Work out the finished part from the listing and answer in its coordinate system (mm). A direction names the side the tool comes from. Give positions to 0.01 mm unless a question says otherwise; leave off trailing zeros. Loops run counter-clockwise (first coordinate to the right, second up) from the corner with the lowest first, then second, coordinate; pieces in that order, holes last. Notation, with made-up numbers: (-6, 69) - (20, 69) arc R25 cw to (20, 81) - close; hole circle Ø8 at (-39.5, -10.75). An arc over 180 degrees is marked (long way). One line per question, with ' | ' between items.
Autodesk Inventor part; units mm, degrees
ref_plane "YZ Plane" through (0, 0, 0) normal (1, 0, 0) x (0, 1, 0)
ref_plane "XZ Plane" through (0, 0, 0) normal (0, 1, 0) x (-1, 0, 0)
ref_plane "XY Plane" through (0, 0, 0) normal (0, 0, 1) x (1, 0, 0)
sketch "Sketch1" plane through (0, 0, 0) normal (0, 0, 1) x (1, 0, 0)
  line L0 (90.4273, 0.002) -> (0, 0.002)
  line L1 (0, 0.002) -> (0, -88.6441)
  arc A0 (0, -88.6441) -> (7.9382, -98.4293) centre (10, -88.6441) ccw
  arc A1 (16.0457, -111.012) -> (7.9382, -98.4293) centre (6.4076, -108.3189) ccw
  arc A2 (145.7944, -114.2869) -> (148.0953, -110.4201) centre (146.9707, -112.3688) ccw
  circle A3 centre (97.4707, -122.3689) radius 2.25
  circle A4 centre (97.4707, -112.3689) radius 2.25
  circle A5 centre (78.1758, -122.3689) radius 2.25
  arc A6 (145.7944, -124.2869) -> (148.0953, -120.4201) centre (146.9707, -122.3689) ccw
  circle A7 centre (22.6171, -8.5119) radius 2.8
  circle A8 centre (22.6171, -40.5119) radius 2.8
  circle A9 centre (28.6758, -122.3689) radius 2.25
  circle A10 centre (28.6758, -112.3689) radius 2.25
  circle A11 centre (78.1758, -112.3689) radius 2.25
  circle A12 centre (78.9344, -21.998) radius 3.25
  circle A13 centre (10, -90.6616) radius 3.3
  line L2 (73.0605, -128.2915) -> (33.527, -128.2915)
  arc A14 (32.527, -127.2915) -> (33.527, -128.2915) centre (33.527, -127.2915) ccw
  line L3 (32.527, -127.2915) -> (32.527, -107.4915)
  arc A15 (33.527, -106.4915) -> (32.527, -107.4915) centre (33.527, -107.4915) ccw
  line L4 (33.527, -106.4915) -> (73.0605, -106.4915)
  arc A16 (74.0605, -107.4915) -> (73.0605, -106.4915) centre (73.0605, -107.4915) ccw
  line L5 (74.0605, -107.4915) -> (74.0605, -127.2915)
  arc A17 (73.0605, -128.2915) -> (74.0605, -127.2915) centre (73.0605, -127.2915) ccw
  line L6 (142.1195, -128.2915) -> (102.586, -128.2915)
  arc A18 (101.586, -127.2915) -> (102.586, -128.2915) centre (102.586, -127.2915) ccw
  line L7 (101.586, -127.2915) -> (101.586, -107.4915)
  arc A19 (102.586, -106.4915) -> (101.586, -107.4915) centre (102.586, -107.4915) ccw
  line L8 (102.586, -106.4915) -> (142.1195, -106.4915)
  arc A20 (143.1195, -107.4915) -> (142.1195, -106.4915) centre (142.1195, -107.4915) ccw
  line L9 (143.1195, -107.4915) -> (143.1195, -127.2915)
  arc A21 (142.1195, -128.2915) -> (143.1195, -127.2915) centre (142.1195, -127.2915) ccw
  circle A22 centre (146.9707, -112.3688) radius 2.25
  circle A23 centre (146.9707, -122.3689) radius 2.25
  line L10 (28.6758, -112.3689) -> (146.9707, -112.3688) construction
  line L11 (28.6758, -122.3689) -> (146.9707, -122.3689) construction
  circle A24 centre (43.3732, -117.3689) radius 5.9 construction
  circle A25 centre (132.2732, -117.3688) radius 5.9 construction
  circle A26 centre (43.3732, -117.3689) radius 6
  circle A27 centre (132.2732, -117.3688) radius 6
  line L12 (10, -90.6616) -> (176.2125, -90.6616) construction
  circle A28 centre (78.9344, -21.998) radius 6
  circle A29 centre (79.375, -41.275) radius 2.8
  line L13 (0.0516, 0) -> (0, 0)
  line L14 (0, 0) -> (0, -88.6441)
  arc A30 (0, -88.6441) -> (8.2038, -98.4815) centre (10, -88.6441) ccw
  arc A31 (16.1218, -110.6924) -> (8.2038, -98.4815) centre (6.4076, -108.3189) ccw
  arc A32 (16.1218, -110.6924) -> (67.3839, -131.6564) centre (43.3217, -117.3382) ccw
  line L15 (67.3839, -131.6564) -> (108.1595, -131.6564)
  arc A33 (108.1595, -131.6564) -> (117.931, -141.4167) centre (132.2217, -117.3382) ccw
  arc A34 (117.931, -141.4167) -> (160.2733, -117.3688) centre (132.2732, -117.3688) ccw
  line L16 (160.2733, -117.3688) -> (160.2733, -88.8237)
  arc A35 (160.2733, -88.8237) -> (156.504, -81.0021) centre (150.2733, -88.8237) ccw
  line L17 (156.504, -81.0021) -> (134.9366, -63.8213)
  arc A36 (131.3222, -57.7523) -> (134.9366, -63.8213) centre (141.1674, -55.9997) ccw
  arc A37 (131.3222, -57.7523) -> (90.9953, -1.4859) centre (52.2705, -71.825) ccw
  arc A38 (90.9953, -1.4859) -> (85.2079, 0.002) centre (85.2079, -11.998) ccw
  line L18 (85.2079, 0.002) -> (0.0516, 0.002)
  line L19 (0.0516, 0.002) -> (0.0516, 0)
  circle A39 centre (155.0516, -88.6441) radius 3.3
  line L20 (102.586, -106.4915) -> (142.1195, -106.4915)
  arc A40 (143.1195, -107.4915) -> (142.1195, -106.4915) centre (142.1195, -107.4915) ccw
  line L21 (143.1195, -107.4915) -> (143.1195, -127.2915)
  arc A41 (142.1195, -128.2915) -> (143.1195, -127.2915) centre (142.1195, -127.2915) ccw
  line L22 (142.1195, -128.2915) -> (102.586, -128.2915)
  arc A42 (101.586, -127.2915) -> (102.586, -128.2915) centre (102.586, -127.2915) ccw
  line L23 (101.586, -127.2915) -> (101.586, -107.4915)
  arc A43 (102.586, -106.4915) -> (101.586, -107.4915) centre (102.586, -107.4915) ccw
  line L24 (74.0605, -107.4915) -> (74.0605, -127.2915)
  arc A44 (73.0605, -128.2915) -> (74.0605, -127.2915) centre (73.0605, -127.2915) ccw
  line L25 (73.0605, -128.2915) -> (33.527, -128.2915)
  arc A45 (32.527, -127.2915) -> (33.527, -128.2915) centre (33.527, -127.2915) ccw
  line L26 (32.527, -127.2915) -> (32.527, -107.4915)
  arc A46 (33.527, -106.4915) -> (32.527, -107.4915) centre (33.527, -107.4915) ccw
  line L27 (33.527, -106.4915) -> (73.0605, -106.4915)
  arc A47 (74.0605, -107.4915) -> (73.0605, -106.4915) centre (73.0605, -107.4915) ccw
  circle A48 centre (28.6758, -112.3689) radius 2.25
  circle A49 centre (28.6758, -122.3689) radius 2.25
  circle A50 centre (78.1758, -21.998) radius 6
  circle A51 centre (78.1758, -122.3689) radius 2.25
  circle A52 centre (97.4707, -112.3689) radius 2.25
  circle A53 centre (146.9707, -112.3688) radius 2.25
  circle A54 centre (146.9707, -122.3689) radius 2.25
  circle A55 centre (22.6171, -8.5119) radius 2.8
  circle A56 centre (22.6171, -40.5119) radius 2.8
  circle A57 centre (97.4707, -122.3689) radius 2.25
  circle A58 centre (78.1758, -112.3689) radius 2.25
  circle A59 centre (10, -88.6441) radius 3.3
  point P0 (0, 0)
  point P1 (58.8546, -117.3689)
  point P2 (148.0953, -110.4201)
  point P3 (151.6186, -98.07)
  point P4 (85.2079, 0.002)
  point P5 (13.142, -89.6529)
  point P6 (6.858, -89.6529)
  point P7 (78.5551, -27.986)
  point P8 (78.5551, -16.01)
  dimension "d2" = 49.5
  dimension "d3" = 49.5
  dimension "d4" = 49.5
  dimension "d5" = 49.5
  dimension "d6" = 10
  dimension "d7" = 12
  dimension "d8" = 12
  dimension "d9" = 6.6
  dimension "d10" = 10
  dimension "d12" = 10
  dimension "d16" = 12
  dimension "d17" = 5.6
  dimension "d18" = 22
extrude "Extrusion1" add sketch "Sketch1" along normal blind 3.175 contours A38 A37 A36 L17 A35 L16 A34 A33 L15 A32 A1 A0 L1 L0 | A22 A2 | A3 | A4 | A5 | A23 A6 | A9 | A10 | A11 | A13 A59 | A59 A13 | A13 A59 | L2 A14 L3 A15 L4 A16 L5 A17 | L6 A18 L7 A19 L8 A20 L9 A21 | A39
properties part number "Intake Sides V4_bearing" material "Polycarbonate, Clear"
1. Determine the mould class of faces 1 (the flat face through (79, -72, 3.175)), 2 (the cylindrical face through (72.177, -22.135, 1.565)), 3 (the cylindrical face through (2.295, -95.018, 1.565)) for opening direction X: +X half, -X half, draft (parallel to the pull), parting line (faces both ways), or undercut.
Evaluation:
face 1: draft | face 2: undercut | face 3: -X half
2. Which of the six approach directions +Z, -Z, +X, -X, +Y, -Y give full straight-line access (tool end or side, diameter ignored) to faces 4 (the cylindrical face through (112.503, -137.217, 1.565)), 5 (the flat face through (79, -72, 0)), 6 (the cylindrical face through (84.933, -21.861, 1.565))?
Evaluation:
face 4: +Z, -Z, -Y | face 5: -Z, +X, -X, +Y, -Y | face 6: +Z, -Z
3. Consider L1, parallel to Y at x = 71, z = 2.4; L2, parallel to X at y = -112, z = 1.85; L3, parallel to Y at x = 25, z = 1.5. Determine where each line is inside the solid, lowest interval first.
Evaluation:
L1: -131.66 to 0 | L2: 15.84 to 40.69, 46.05 to 129.59, 134.95 to 160.27 | L3: -138.51 to -41.98, -39.04 to -9.98, -7.04 to 0
4. Find section B-B on z = 1.9. Write down the section's boundary in (x, y) (1 decimal).
Evaluation:
outline: (0, -88.6) arc R10 ccw to (7.9, -98.4) arc R10 cw to (16, -111) arc R28 ccw to (67.4, -131.7) - (108.2, -131.7) arc R28 ccw to (117.9, -141.4) arc R28 ccw to (160.3, -117.4) - (160.3, -88.8) arc R10 ccw to (156.5, -81) - (134.9, -63.8) arc R10 cw to (131.3, -57.8) arc R80.3 ccw to (91, -1.5) arc R12 ccw to (85.2, 0) - (0, 0) - close; hole circle Ø5.6 at (22.6, -40.5); hole circle Ø5.6 at (22.6, -8.5); hole circle Ø12 at (43.4, -117.4); hole circle Ø5.6 at (79.4, -41.3); hole (78.6, -28) arc R6 ccw (long way) to (78.6, -16) arc R6 ccw (long way) to start; hole circle Ø12 at (132.3, -117.4)
5. Find section D-D on x = 13. Write down the section's boundary in (y, z) (3 decimals).
Evaluation:
outline: (-100.79, 0) - (0.002, 0) - (0.002, 3.175) - (-100.79, 3.175) - close
6. Flat-ended cylindrical pins translate along their axes: pin 1 (4.5 mm diameter, centred on x = 22.62, y = -40.51, fed in from +Z); pin 2 (1 mm diameter, centred on y = -119.5, z = 2.5, fed in from -X); pin 3 (1 mm diameter, centred on x = 91, z = 1.5, fed in from +Y). Find the tip coordinate at first contact, or state that the pin passes through.
Evaluation:
pin 1: through | pin 2: x = 15.37 | pin 3: y = -1.23
7. Find section C-C on y = -62. Write down the section's boundary in (x, z) (3 decimals).
Evaluation:
outline: (0, 0) - (133.168, 0) - (133.168, 3.175) - (0, 3.175) - close
8. Find section A-A on x = 42. Write down the section's boundary in (y, z) (3 decimals).
Evaluation:
outline: (-145.307, 0) - (-123.21, 0) - (-123.21, 3.175) - (-145.307, 3.175) - close; (-111.528, 0) - (0.002, 0) - (0.002, 3.175) - (-111.528, 3.175) - close
